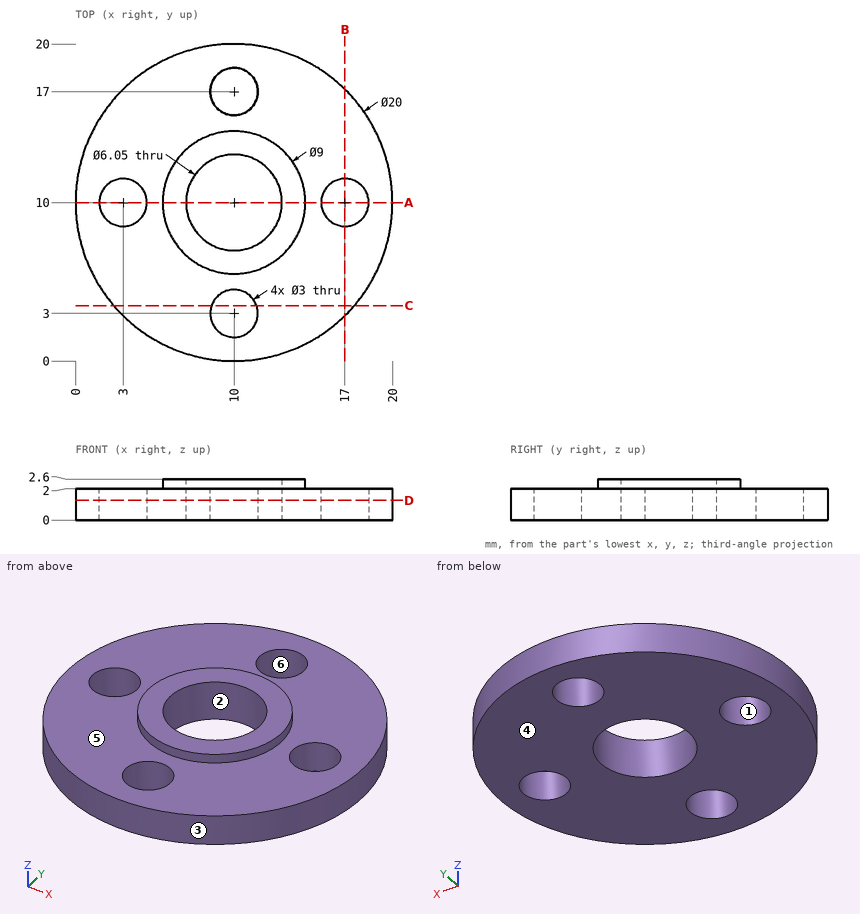
Input: dimensioned drawing with shaded views. Units: mm. Origin: part minimum x, y, z. A direction names the side the tool comes from. Round coordinates to 2 decimals unless told otherwise and drop trailing zeros. Loops run counter-clockwise (first coordinate to the right, second up) from the corner with the lowest first, then second, coordinate; pieces in that order, holes last. Notation, with made-up numbers: (85.25, 8.25) -> (138.25, 8.25) arc R26 ccw to (138.25, 47.25) -> close; hole circle Ø3 at (53.25, -10.75). An arc over 180 degrees is marked (long way). Answer as a JSON object with one key per item and string values. Group by question number.
Q1. Ray query, line 1 (Y direction, x = 10, z = 0.4) (3 decimals); line 2 (X direction, y = 8.75, z = 1.1). Return the intervals inside material, ascending. Write a range as from..to.
Q2. Contact query for flat-ended pins moving along their axis: P1, Ø1.5, axis at x = 10, y = 16, coming from the +Z side; P2, Ø1, axis at x = 14, z = 2, coming from the -Y side. Output: stop coordinate, or through.
Q3. Section query A-A (y = 10). Output: boundary loops of the cut face in (x, z) (3 decimals).
Q4. Section query C-C (y = 3.5). Output: boundary loops of the cut face in (x, z), plus the area to 3 significant figures.
Q5. Access query for the marked faces 5 and 6. Directions: +Z, -Z, +X, -X, +Y, -Y. A direction counts if a zero-diameter tool reaches every point of the face in a straight line with its end or side. Return the directions, or none.
Q6. Section query B-B (x = 17). Output: boundary loops of the cut face in (y, z).
Q7. Mould query, pull axis X, two halves, no side actions, for the marked faces 1, 2, 3 and 4. Classes: pulls with the +X half, pulls with the -X half, needs draft (parallel to the pull), parting line crosses it, or undercut.
Q8. Section query D-D (z = 1.25). Output: boundary loops of the cut face in (x, y) (3 decimals), plus the area to 3 significant figures.
Completed:
{
 "1": {"line 1": "0..1.5, 4.5..6.975, 13.025..15.5, 18.5..20", "line 2": "0.08..2.17, 3.83..7.25, 12.75..16.17, 17.83..19.92"},
 "2": {"P1": "z = 2", "P2": "y = 0.63"},
 "3": {"outline": "(0, 0) -> (1.5, 0) -> (1.5, 2) -> (0, 2) -> close; (4.5, 0) -> (6.975, 0) -> (6.975, 2.6) -> (5.5, 2.6) -> (5.5, 2) -> (4.5, 2) -> close; (13.025, 0) -> (15.5, 0) -> (15.5, 2) -> (14.5, 2) -> (14.5, 2.6) -> (13.025, 2.6) -> close; (18.5, 0) -> (20, 0) -> (20, 2) -> (18.5, 2) -> close"},
 "4": {"outline": "(2.4, 0) -> (8.59, 0) -> (8.59, 2) -> (2.4, 2) -> close; (11.41, 0) -> (17.6, 0) -> (17.6, 2) -> (11.41, 2) -> close", "area": "24.7 mm²"},
 "5": {"face 5": "+Z", "face 6": "+Z, -Z"},
 "6": {"outline": "(2.86, 0) -> (8.5, 0) -> (8.5, 2) -> (2.86, 2) -> close; (11.5, 0) -> (17.14, 0) -> (17.14, 2) -> (11.5, 2) -> close"},
 "7": {"face 1": "undercut", "face 2": "undercut", "face 3": "parting line crosses it", "face 4": "needs draft"},
 "8": {"outline": "circle Ø20 at (10, 10); hole circle Ø3 at (3, 10); hole circle Ø6.05 at (10, 10); hole circle Ø3 at (10, 3); hole circle Ø3 at (10, 17); hole circle Ø3 at (17, 10)", "area": "257 mm²"}
}
